Source: CAD feature listing. Evaluate the final solid. Frame: model axes, mm. A direction names the side the tool comes from. Round coordinates to 2 decimals unless told otherwise and drop trailing zeros. Loops run counter-clockwise (first coordinate to the right, second up) from the corner with the lowest first, then second, coordinate; pieces in that order, holes last.
Item 1: First-contact query: P1, Ø7, axis at y = 0.33, z = 30, coming from the -X side; P2, Ø3.5, axis at y = 8.96, z = 44.94, coming from the +X side. Flat tips, straight axial feed; report the tip coordinate or a pass-through.
Item 2: Ray query, L1, parallel to Y at x = 93, z = 30; L2, parallel to X at y = 4, z = 57; L3, parallel to X at y = -78.4, z = 30. Return the intervals inside material, ascending.
Item 3: Pull-direction query (Z, two-part tool) for faces 1 (the flat face through (45, -79, 0)), 2 (the flat face through (-2, 48.163, 30)), 3 (the cylindrical face through (92.46, -8.21, 13.06)); classes: released by +Z, released by -Z, zero draft, split by the parting line, or undercut.
Item 4: Access query for faces 4 (the cylindrical face through (-2.465, -2.103, 33.174)), 5 (the cylindrical face through (92.46, -8.21, 42.94)), 6 (the flat face through (46, -76.837, 30)). Directions: +Z, -Z, +X, -X, +Y, -Y. A direction counts if a zero-diameter tool reaches every point of the face in a straight line with its end or side. Return the directions, or none.
Item 5: Section query D-D on x = 20. Return loops of the section in (y, z), then the cut area to 3 significant figures.
Item 6: Section query C-C on z = 24. Return loops of the section in (x, y).
Item 7: Section query A-A on y = -43.5. Return loops of the section in (x, z), then the cut area to 3 significant figures.
Item 8: Section query B-B on x = 3. Return loops of the section in (y, z), then the cut area to 3 significant figures.
```python
from build123d import *

# Parameters (mm, degrees)
EXTRUDE_1_DEPTH     = 60
SKETCH_2_R          = 2
CUT_EXTRUDE_1_DEPTH = 6
SKETCH_3_R          = 2
SKETCH_3_R_2        = 0.32384185
CUT_EXTRUDE_2_DEPTH = 10
SKETCH_5_R          = 4
SKETCH_5_R_2        = 0.32384185
CUT_EXTRUDE_4_DEPTH = 6


with BuildPart() as part:
    # 草图1 → 凸台-拉伸1 (new body)
    with BuildSketch(Plane.XY):
        Polygon((95, -81.837278389), (95, 48.162721611), (90, 48.162721611), (90, -76.837278389), (0, -76.837278389), (0, 48.162721611), (-5, 48.162721611), (-5, -81.837278389), align=None)
    extrude(amount=EXTRUDE_1_DEPTH)

    # 草图2 → 切除-拉伸1 (cut, through all)
    with BuildSketch(Plane(origin=(0, -76.837278389, 0), x_dir=(1, 0, 0), z_dir=(0, 1, 0))):
        with Locations((3, -30)):
            Circle(SKETCH_2_R)
        with Locations((87, -30)):
            Circle(SKETCH_2_R)
    extrude(amount=-CUT_EXTRUDE_1_DEPTH, mode=Mode.SUBTRACT)

    # 草图3 → 切除-拉伸2 (cut)
    with BuildSketch(Plane.ZY.offset(-90)):
        with Locations((30, 17.582413023)):
            Circle(SKETCH_3_R)
        with Locations((15.060150537, 8.956886914)):
            Circle(SKETCH_3_R)
        with Locations((15.060150537, -8.294165304)):
            Circle(SKETCH_3_R)
        with Locations((30, -16.919691412)):
            Circle(SKETCH_3_R)
        with Locations((44.939849463, -8.294165304)):
            Circle(SKETCH_3_R)
        with Locations((44.939849463, 8.956886914)):
            Circle(SKETCH_3_R)
        with Locations((30, 0.331360805)):
            Circle(SKETCH_3_R_2)
    extrude(amount=-CUT_EXTRUDE_2_DEPTH, mode=Mode.SUBTRACT)

    # 草图5 → 切除-拉伸4 (cut, through all)
    with BuildSketch(Plane(origin=(0, 0, 0), x_dir=(0, 0, -1), z_dir=(1, 0, 0))):
        with Locations((-30, 0.331360805)):
            Circle(SKETCH_5_R)
        with Locations((-30, 0.331360805)):
            Circle(SKETCH_5_R_2, mode=Mode.SUBTRACT)
        with Locations((-30, 0.331360805)):
            Circle(SKETCH_5_R_2)
    extrude(amount=-CUT_EXTRUDE_4_DEPTH, mode=Mode.SUBTRACT)


solid = part.part
```
Data:
1. P1: stops at x = 90
1. P2: stops at x = 0
2. L1: y = -81.84 to -18.92, -14.92 to 0.01, 0.66 to 15.58, 19.58 to 48.16
2. L2: x = -5 to 0, 90 to 95
2. L3: x = -5 to 1, 5 to 85, 89 to 95
3. face 1: released by -Z
3. face 2: zero draft
3. face 3: undercut
4. face 4: -X
4. face 5: +X
4. face 6: +Z, -Z, +Y
5. outline: (-81.84, 0) - (-76.84, 0) - (-76.84, 60) - (-81.84, 60) - close
5. area: 300 mm2
6. outline: (-5, -81.84) - (95, -81.84) - (95, 48.16) - (90, 48.16) - (90, -76.84) - (0, -76.84) - (0, 48.16) - (-5, 48.16) - close
7. outline: (-5, 0) - (0, 0) - (0, 60) - (-5, 60) - close; (90, 0) - (95, 0) - (95, 60) - (90, 60) - close
7. area: 600 mm2
8. outline: (-81.84, 0) - (-76.84, 0) - (-76.84, 28) - (-81.84, 28) - close; (-81.84, 32) - (-76.84, 32) - (-76.84, 60) - (-81.84, 60) - close
8. area: 280 mm2
